Here's how the part is built. I have some questions about the finished solid (model axes, mm). Give positions to 0.01 mm unless a question says otherwise; leave off trailing zeros. Loops run counter-clockwise (first coordinate to the right, second up) from the corner with the lowest first, then second, coordinate; pieces in that order, holes last. Notation, with made-up numbers: (48.25, -22.5) - (63.25, -22.5) arc R20 ccw to (63.25, -11.5) - close; hole circle Ø7 at (61, -25.5). An arc over 180 degrees is marked (long way). Use a Markdown table: item, result.
from build123d import *

# Parameters (mm, degrees)
SKETCH_1_R      = 1.6
EXTRUDE_1_DEPTH = 3


with BuildPart() as part:
    # 草图1 → 凸台-拉伸1 (new body)
    with BuildSketch(Plane(origin=(0, 0, 0), x_dir=(1, 0, 0), z_dir=(0, 1, 0))):
        with BuildLine():
            Line((-80.009028181, 21.402670377), (-80.009028181, -28.604431477))
            ThreePointArc((-80.009028181, -28.604431477), (-79.134066788, -30.716775138), (-77.021723127, -31.591736531))
            Line((-77.021723127, -31.591736531), (12.787258331, -31.591736531))
            ThreePointArc((12.787258331, -31.591736531), (14.899601993, -30.716775138), (15.774563386, -28.604431477))
            Line((15.774563386, -28.604431477), (15.774563386, 21.402670377))
            ThreePointArc((15.774563386, 21.402670377), (14.899601993, 23.515014039), (12.787258331, 24.389975432))
            Line((12.787258331, 24.389975432), (-77.021723127, 24.389975432))
            ThreePointArc((-77.021723127, 24.389975432), (-79.134066788, 23.515014039), (-80.009028181, 21.402670377))
        make_face()
        with Locations(Location((-76.52848462, 20.886724226, 0), (0, 0, 270))):
            Circle(SKETCH_1_R, mode=Mode.SUBTRACT)
        with Locations(Location((-18.52858622, 20.886597225, 0), (0, 0, 270))):
            Circle(SKETCH_1_R, mode=Mode.SUBTRACT)
        with Locations(Location((-18.52833222, -28.113656775, 0), (0, 0, 270))):
            Circle(SKETCH_1_R, mode=Mode.SUBTRACT)
        with Locations(Location((-76.52833222, -28.113529775, 0), (0, 0, 270))):
            Circle(SKETCH_1_R, mode=Mode.SUBTRACT)
        with BuildLine():
            Line((-70.903401709, 18.230282987), (-54.564490165, 18.082300473))
            ThreePointArc((-54.564490165, 18.082300473), (-53.860065027, 17.78301522), (-53.573587867, 17.073284796))
            Line((-53.573587867, 17.073284796), (-53.940568984, -23.445502526))
            ThreePointArc((-53.940568984, -23.445502526), (-54.239854236, -24.149927664), (-54.94958466, -24.436404824))
            Line((-54.94958466, -24.436404824), (-71.288496204, -24.288422311))
            ThreePointArc((-71.288496204, -24.288422311), (-71.992921342, -23.989137058), (-72.279398502, -23.279406634))
            Line((-72.279398502, -23.279406634), (-71.912417386, 17.239380688))
            ThreePointArc((-71.912417386, 17.239380688), (-71.613132133, 17.943805826), (-70.903401709, 18.230282987))
        make_face(mode=Mode.SUBTRACT)
    extrude(amount=EXTRUDE_1_DEPTH)


solid = part.part
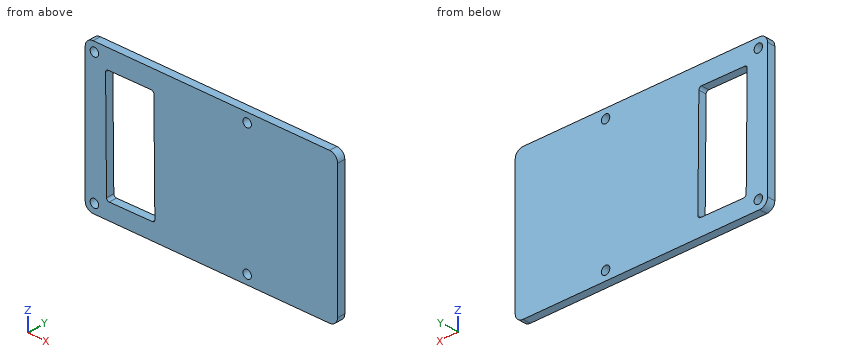
(1) If I drill on line 1 (X direction, y = 0.7, z = 23.5); line 2 (Z direction, x = -75.5, y = 2.35); line 3 (X direction, y = 1.3, z = 0), over which ranges is the centre line in solid material (lowest first)?
A:
| item | result |
|---|---|
| line 1 | -80.01 to -72.26, -53.94 to 15.77 |
| line 2 | -24.39 to -22.11, -19.66 to 26.89, 29.34 to 31.59 |
| line 3 | -80.01 to -72.07, -53.73 to 15.77 |
(2) Suppose I cut it at C-C on y = 1.2. Write out the boundary of the cut face in (x, z), plus the area to 3 significant figures.
A:
| item | result |
|---|---|
| outline | (-80.01, -21.4) arc R2.99 ccw to (-77.02, -24.39) - (12.79, -24.39) arc R2.99 ccw to (15.77, -21.4) - (15.77, 28.6) arc R2.99 ccw to (12.79, 31.59) - (-77.02, 31.59) arc R2.99 ccw to (-80.01, 28.6) - close; hole circle Ø3.2 at (-76.53, -20.89); hole circle Ø3.2 at (-76.53, 28.11); hole (-72.28, 23.28) - (-71.91, -17.24) arc R1 ccw to (-70.9, -18.23) - (-54.56, -18.08) arc R1 ccw to (-53.57, -17.07) - (-53.94, 23.45) arc R1 ccw to (-54.95, 24.44) - (-71.29, 24.29) arc R1 ccw to start; hole circle Ø3.2 at (-18.53, -20.89); hole circle Ø3.2 at (-18.53, 28.11) |
| area | 4,540 mm2 |
(3) Suppose I cut it at B-B on z = 8.5. Write out the boundary of the cut face in (x, y).
A:
| item | result |
|---|---|
| outline | (-80.01, 0) - (-72.15, 0) - (-72.15, 3) - (-80.01, 3) - close; (-53.81, 0) - (15.77, 0) - (15.77, 3) - (-53.81, 3) - close |
(4) Suppose I cut it at A-A on x = -58.5. Write out the boundary of the cut face in (y, z).
A:
| item | result |
|---|---|
| outline | (0, -24.39) - (3, -24.39) - (3, -18.12) - (0, -18.12) - close; (0, 24.4) - (3, 24.4) - (3, 31.59) - (0, 31.59) - close |
(5) Will this pin go through, and if not, where does the flat tip stop? pin 1 (3 mm diameter, centred on x = -18.53, z = -20.89, fed in from +Y).
A:
| item | result |
|---|---|
| pin 1 | through |
